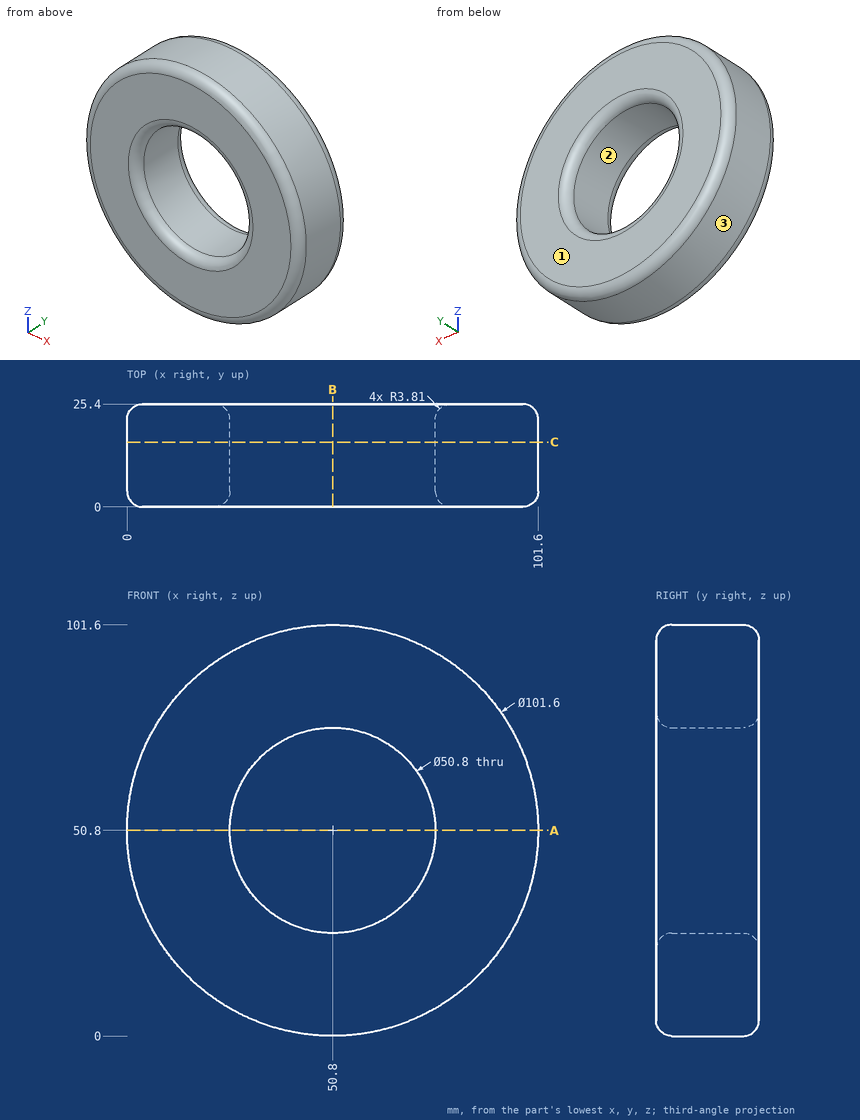
Drawing for the job (mm, zero at the part's lowest x, y, z). Give positions to 0.01 mm unless a question says otherwise; leave off trailing zeros. Write each loop counter-clockwise with the first axis right and the second up, starting at its lowest first coordinate (ties: lowest second). Pieces come first, ordered by that corner, then holes. Notation, with made-up numbers: M 12,58 L 53,58 A20 ccw 53,85 Z; hole C 24,65 d2. An arc over 180 degrees is marked long. Return JSON: item names as keys, results as strings. Group by question number.
(1) Band-saw the part on C-C (y = 16). Give the cut face in (x, z), and give its area (3 significant figures).
(2) Flat gauge pins, fed straight in: pin 1 Ø12 at (x, y) = (17, 3.5) entering from -Z; pin 2 Ø12 at (y, z) = (6.5, 65) entering from -X; pin 3 Ø5 at (y, z) = (22.5, 14.5) entering from +X. Where does each tip first touch, or does it go through?
(3) Band-saw the part on A-A (z = 50.8). Give the cut face in (x, y), and give its area (3 significant figures).
(4) Mould opens along Z. For the marked faces 1, 2 and 3 say: pulls with the +Z half, pulls with the -Z half, needs draft (parallel to the pull), parting line crosses it, or undercut.
(5) Drill centre lines: L1, parallel to X at y = 14, z = 50.8; L2, parallel to X at y = 12, z = 59; L3, parallel to Z at x = 56, y = 18. Where is each one in solid material? Low to high. Write a range as [from, to].
(6) Band-saw the part on B-B (x = 50.8). Give the cut face in (y, z).
Entries:
{
 "1": {"outline": "C 50.8,50.8 d101.6; hole C 50.8,50.8 d50.8", "area": "6,080 mm^2"},
 "2": {"pin 1": "stops at z = 8.29", "pin 2": "stops at x = 0.67", "pin 3": "stops at x = 88.65"},
 "3": {"outline": "M 0,3.81 A3.81 ccw 3.81,0 L 21.59,0 A3.81 ccw 25.4,3.81 L 25.4,21.59 A3.81 ccw 21.59,25.4 L 3.81,25.4 A3.81 ccw 0,21.59 Z; M 76.2,3.81 A3.81 ccw 80.01,0 L 97.79,0 A3.81 ccw 101.6,3.81 L 101.6,21.59 A3.81 ccw 97.79,25.4 L 80.01,25.4 A3.81 ccw 76.2,21.59 Z", "area": "1,270 mm^2"},
 "4": {"face 1": "needs draft", "face 2": "undercut", "face 3": "parting line crosses it"},
 "5": {"L1": "x = [0, 25.4], [76.2, 101.6]", "L2": "x = [0.67, 26.76], [74.84, 100.93]", "L3": "z = [0.27, 25.94], [75.66, 101.33]"},
 "6": {"outline": "M 0,3.81 A3.81 ccw 3.81,0 L 21.59,0 A3.81 ccw 25.4,3.81 L 25.4,21.59 A3.81 ccw 21.59,25.4 L 3.81,25.4 A3.81 ccw 0,21.59 Z; M 0,80.01 A3.81 ccw 3.81,76.2 L 21.59,76.2 A3.81 ccw 25.4,80.01 L 25.4,97.79 A3.81 ccw 21.59,101.6 L 3.81,101.6 A3.81 ccw 0,97.79 Z"}
}
